from build123d import *

# Parameters (mm, degrees)
SKETCH1_R           = 1.75
BOSS_EXTRUDE1_DEPTH = 5


with BuildPart() as part:
    # Sketch1 → Boss-Extrude1 (new body)
    with BuildSketch(Plane.XY):
        with BuildLine():
            Line((-9.5, -179.270297721), (-9.5, -6.429702279))
            ThreePointArc((-9.5, -6.429702279), (-8.914213562, -5.015488716), (-7.5, -4.429702279))
            Line((-7.5, -4.429702279), (7.5, -4.429702279))
            ThreePointArc((7.5, -4.429702279), (8.914213562, -5.015488716), (9.5, -6.429702279))
            Line((9.5, -6.429702279), (9.5, -179.270297721))
            ThreePointArc((9.5, -179.270297721), (8.914213562, -180.684511284), (7.5, -181.270297721))
            Line((7.5, -181.270297721), (-7.5, -181.270297721))
            ThreePointArc((-7.5, -181.270297721), (-8.914213562, -180.684511284), (-9.5, -179.270297721))
        make_face()
        with Locations((5, -8.429702279)):
            Circle(SKETCH1_R, mode=Mode.SUBTRACT)
        with Locations((-5, -8.429702279)):
            Circle(SKETCH1_R, mode=Mode.SUBTRACT)
        with Locations(Location((-5, -177.270297721, 0), (0, 0, 180))):
            Circle(SKETCH1_R, mode=Mode.SUBTRACT)
        with Locations(Location((5, -177.270297721, 0), (0, 0, 180))):
            Circle(SKETCH1_R, mode=Mode.SUBTRACT)
    extrude(amount=BOSS_EXTRUDE1_DEPTH)


solid = part.part
Part model, mm, in its own coordinate system. Give positions to 0.01 mm unless a question says otherwise; leave off trailing zeros. Loops run counter-clockwise (first coordinate to the right, second up) from the corner with the lowest first, then second, coordinate; pieces in that order, holes last. Notation, with made-up numbers: (56, 16) -> (65, 16) arc R26 ccw to (65, 45) -> close; hole circle Ø7 at (-23, -31.75). An arc over 180 degrees is marked (long way). Write each question's results on one line, items separated by ' | '. Start each with the question number.
Q1. Pull direction Z, two halves, no side cores. Call faces 1 (the face through (3.25, -8.35, 2.46)), 2 (the face through (0, -92, 5)), 3 (the face through (0, -92, 0)): +Z half, -Z half, draft (parallel to the pull), parting line (faces both ways), or undercut.
Q2. Pin check, flat tip, straight feed: P1, Ø3, axis at x = 5, y = -177.27, coming from the +Z side. Stop position of the tip, or through.
Q3. Band-saw the part on A-A on x = -5. List the corners of the cut face in (y, z), plus the area to 3 significant figures.
Q4. Wall check: L1, parallel to Y at x = -4.75, z = 2.5; L2, parallel to Y at x = 6, z = 0.65; L3, parallel to Y at x = -7.75, z = 0.9. Give the ranges that are in metal, low to high.
Results are:
1) face 1: draft | face 2: +Z half | face 3: -Z half
2) P1: passes through
3) outline: (-181.27, 0) -> (-179.02, 0) -> (-179.02, 5) -> (-181.27, 5) -> close; (-175.52, 0) -> (-10.18, 0) -> (-10.18, 5) -> (-175.52, 5) -> close; (-6.68, 0) -> (-4.43, 0) -> (-4.43, 5) -> (-6.68, 5) -> close | area: 849 mm²
4) L1: y = -181.27 to -179, -175.54 to -10.16, -6.7 to -4.43 | L2: y = -181.27 to -178.71, -175.83 to -9.87, -6.99 to -4.43 | L3: y = -181.25 to -4.45
